The listing builds one solid part. Answer for the finished solid, in the listing's coordinates (mm). A direction names the side the tool comes from. Coordinates: 2 decimals unless noted, no trailing zeros. Order: outer loops, then holes, each group sorted by start corner. A loop starts at its lowest first (then second) coordinate and runs counter-clockwise, first axis right, second up. Notation, with made-up numbers: (87, -15.75) -> (113, -15.75) arc R23 cw to (113, 0.25) -> close; hole circle Ø6 at (49.5, 75). An arc over 180 degrees is marked (long way). Return JSON: item names as keys, results as strings.
from build123d import *


with BuildPart() as part:
    # Sketch_plunger → Rev_plunger (revolve)
    with BuildSketch(Plane(origin=(0, 0, 0), x_dir=(1, 0, 0), z_dir=(0, 1, 0)), mode=Mode.PRIVATE) as rev_plunger_sk:
        with BuildLine():
            Line((0, 5), (0, -24))
            Line((0, -24), (4, -24))
            Line((4, -24), (4, -18))
            Line((4, -18), (6, -18))
            Line((6, -18), (6, -10.4))
            Line((6, -10.4), (4.3, -10.4))
            Line((4.3, -10.4), (4.3, -8))
            Line((4.3, -8), (6, -8))
            Line((6, -8), (6, 0))
            Line((6, 0), (5, 0))
            ThreePointArc((5, 0), (3.5355, 3.5355), (0, 5))
        make_face()
    revolve(rev_plunger_sk.sketch.rotate(Axis((0, 0, 0), (0, 0, 1)), 180), axis=Axis((0, 0, 0), (0, 0, 1)))

    # Chamfer_C05: read off the stored shape, not the designer's step
    # Chamfer_C05 outline → Chamfer_C05 (revolve, cut)
    with BuildSketch(Plane.XZ):
        Polygon((3.5, 24), (4, 23.5), (4, 24), align=None)
        Polygon((6, 18), (5.5, 18), (6, 17.5), align=None)
        Polygon((6, -0.52796442), (6, 0.5), (5.5, 0), (5.5, -0.52796442), align=None)
    revolve(axis=Axis((0, 0, 0), (0, 0, 1)), mode=Mode.SUBTRACT)

    # Chamfer_C05 2 outline → Chamfer_C05 2 (revolve)
    with BuildSketch(Plane.XZ):
        Polygon((4.5, 18), (4, 18.5), (4, 18), align=None)
        Polygon((5.5, 0.5), (4.97203558, 0.5), (4.97203558, -0.52796442), (5.5, 0), align=None)
    revolve(axis=Axis((0, 0, 0), (0, 0, 1)))

    # Chamfer_C05 3 outline → Chamfer_C05 3 (revolve)
    with BuildSketch(Plane.XZ):
        Polygon((5.5, 0.5), (5.5, 0), (6, 0.5), align=None)
    revolve(axis=Axis((0, 0, 0), (0, 0, 1)))


solid = part.part
1. The part is cut by section A-A on z = 22. Give the vertices of the cut face in (x, y), and give its area (3 significant figures).
Answer block:
{"outline": "circle Ø8 at (0, 0)", "area": "50.3 mm2"}
2. Consider line 1 (Z direction, x = 5, y = 0.75); line 2 (Y direction, x = -0.25, z = 16.25); line 3 (Z direction, x = 0, y = 5). Determine where each line is inside the solid, lowest interval first. Write a range as from..to.
Answer block:
{"line 1": "z = -0.44..8, 10.4..18", "line 2": "y = -5.99..5.99", "line 3": "z = -0.5..8, 10.4..18"}
3. The part is cut by section B-B on z = 11.5. Give the vertices of the cut face in (x, y), and give its area (3 significant figures).
Answer block:
{"outline": "circle Ø12 at (0, 0)", "area": "113 mm2"}
4. Each of these flat-tipped pins is pushed along its axis until it touches: pin 1 Ø6 at (y, z) = (4.5, 14) entering from +X; pin 2 Ø1.5 at (y, z) = (2.5, 9.5) entering from +X; pin 3 Ø4 at (x, y) = (1, 2) entering from -Z. Where does it stop, or does it pass through?
Answer block:
{"pin 1": "stops at x = 5.81", "pin 2": "stops at x = 3.93", "pin 3": "stops at z = -4.99"}
5. Determine the mould class of faces 1 (the face through (-3, 4, 10.4)), 2 (the face through (0, 0, 24)), 3 (the face through (0.867, 3.905, 20.965)) for opening direction Z: pulls with the +Z half, pulls with the -Z half, needs draft (parallel to the pull), parting line crosses it, or undercut.
Answer block:
{"face 1": "undercut", "face 2": "pulls with the +Z half", "face 3": "needs draft"}
6. For faces 4 (the face through (4.296, -0.189, 9.183)), 5 (the face through (-5, 0, 18)), 6 (the face through (-5.723, -1.802, 4.198)), determine the directions among +Z, -Z, +X, -X, +Y, -Y from which every point of the face is accessible in a straight line to the end or side of a thin tool.
Answer block:
{"face 4": "none", "face 5": "+Z", "face 6": "+Z, -Z"}
